Autodesk Fusion 360 part; units mm, degrees
sketch "rectangle" plane through (0, 0, 0) normal (0, 0, 1) x (1, 0, 0)
  line L0 (70, 35) -> (-70, 35)
  line L1 (-70, 35) -> (-70, -35)
  line L2 (-70, -35) -> (70, -35)
  line L3 (70, -35) -> (70, 35)
  line L4 (70, 35) -> (-70, -35) construction
  line L5 (-70, 35) -> (70, -35) construction
  dimension "d1" = 70
  dimension "d2" = 140
extrude "Extrude1" add sketch "rectangle" along normal blind 8
sketch "Sketch2" plane through (0, 0, 0) normal (0, 0, -1) x (1, 0, 0)
  line L0 (70, -35) -> (70, 35)
  line L1 (70, 35) -> (-70, 35)
  line L2 (-70, 35) -> (-70, -35)
  line L3 (-70, -35) -> (70, -35)
  line L4 (10, -45) -> (-10, -45)
  line L5 (-10, -45) -> (-10, 45)
  line L6 (-10, 45) -> (10, 45)
  line L7 (10, 45) -> (10, -45)
  line L8 (-6, 39) -> (-6, 21.0153)
  arc A0 (-6, 21.0153) -> (6, 21.0153) centre (0, 21.0153) ccw
  line L9 (6, 21.0153) -> (6, 39)
  arc A1 (6, 39) -> (-6, 39) centre (0, 39) ccw
  line L10 (0, 45) -> (0, 15.0153) construction
  dimension "d5" = 90
  dimension "d8" = 12
extrude "Extrude2" add sketch "Sketch2" along normal blind 8 contours L3 L4 L5 L7 | L1 L3 L5 L7 L8 A0 L9 | L1 L6 L7 L9 A1 | L1 L8 A0 L9 | L1 L8 L9 A1 | L1 L5 L6 L8 A1
sketch "Sketch3" plane through (0, 0, -8) normal (0, 0, -1) x (1, 0, 0)
  line L0 (10, 45) -> (-10, 45)
  line L1 (-10, 45) -> (-10, -45)
  line L2 (-10, -45) -> (10, -45)
  line L3 (10, -45) -> (10, 45)
  line L4 (10, -30) -> (10, 30)
  arc A0 (10, 30) -> (-10, 30) centre (0, 30) ccw
  line L5 (-10, 30) -> (-10, -30)
  arc A1 (-10, -30) -> (10, -30) centre (0, -30) ccw
  line L6 (0, -30) -> (0, 30) construction
extrude "Extrude3" add sketch "Sketch3" along normal blind 8 contours L1 L3 L4 A0 L5 A1
sketch "Sketch4" plane through (0, 0, -8) normal (0, 0, -1) x (1, 0, 0)
  arc A0 (-10, -30) -> (10, -30) centre (0, -30) ccw
  line L0 (-10, -45) -> (10, -45)
hole "Hole1" at (0, -30, -16) direction (0, 0, 1) diameter 10 depth 20 tip angle 118
hole "Hole2" at (0, 30, -16) direction (0, 0, 1) diameter 10 depth 20 tip angle 118
hole "Hole3" at (0, 0, -16) direction (0, 0, 1) diameter 10 depth 20 tip angle 118
fillet "Fillet1" radius 2 3 edges at (-10, -37.5, -8) (-10, -45, -4) (0, -45, -8)
fillet "Fillet2" radius 2 3 edges at (10, -45, -3) (10, -44.4142, -7.4142) (10, -36.5, -8)
fillet "Fillet3" radius 2 2 edges at (-10, 37.5, -8) (-10, 45, -4)
fillet "Fillet4" radius 2 2 edges at (10, 37.5, -8) (10, 45, -4)
Read the model definition and answer for the solid it produces. Units are mm, in the model's axes. A direction names the side the tool comes from. Round coordinates to 2 decimals unless told otherwise and drop trailing zeros. Write each loop counter-clockwise with the first axis right and the second up, starting at its lowest first coordinate (ties: lowest second). Pieces come first, ordered by that corner, then holes. Notation, with made-up numbers: (-39.75, 26) -> (-31.75, 26) arc R25 cw to (-31.75, 61) -> close; hole circle Ø10 at (23.25, 16). An arc over 180 degrees is marked (long way). Answer in a Markdown table with one row per item. Add a question column.
1) Find section A-A, the plane z = -11.5. Determine the outline of the cut face in (x, y), and give its area (3 significant figures).
2) Determine the mould class of faces 4 (the face through (-70, 0, 4)), 5 (the face through (0.04, -30.87, 6.48)), 6 (the face through (-7, -1, -16)) for opening direction X: pulls with the +X half, pulls with the -X half, needs draft (parallel to the pull), parting line crosses it, or undercut.
3) Given P1, Ø18, axis at x = -41, y = -16, coming from the -Z side; P2, Ø6.5, axis at x = 20, z = 2.5, coming from the -Y side; P3, Ø2.5, axis at x = 3.5, y = 40.5, coming from the -Z side; P4, Ø5, axis at y = -27, z = -7, coming from the -X side, each flat-ended and moving along its own axis, determine where each tip first touches the part or whether it passes through.
4) Find section B-B, the plane y = 21. Determine the outline of the cut face in (x, z).
5) Which of the six approach directions +Z, -Z, +X, -X, +Y, -Y give full straight-line access (tool end or side, diameter ignored) to faces 1 (the face through (0, -40, 0)), 2 (the face through (0, 40, 0)), 3 (the face through (0, -40, -12))?
6) Consider line 1 (Y direction, x = 0, z = -11.25); line 2 (Y direction, x = 0, z = -3); line 3 (X direction, y = -30, z = -8). Determine where each line is inside the solid, lowest interval first.
7) Find section D-D, the plane z = 2. Determine the outline of the cut face in (x, y), and give its area (3 significant figures).
8) Find section C-C, the plane x = 45.5. Determine the outline of the cut face in (y, z), and give its area (3 significant figures).
Findings below:
| question | item | result |
|---|---|---|
| 1 | outline | (-10, -30) arc R10 ccw to (10, -30) -> (10, 30) arc R10 ccw to (-10, 30) -> close; hole circle Ø10 at (0, -30); hole circle Ø10 at (0, 0); hole circle Ø10 at (0, 30) |
| 1 | area | 1,280 mm² |
| 2 | face 4 | pulls with the -X half |
| 2 | face 5 | undercut |
| 2 | face 6 | needs draft |
| 3 | P1 | z = 0 |
| 3 | P2 | y = -35 |
| 3 | P3 | z = -16 |
| 3 | P4 | x = -10 |
| 4 | outline | (-70, 0) -> (-10, 0) -> (-10, -16) -> (10, -16) -> (10, 0) -> (70, 0) -> (70, 8) -> (-70, 8) -> close |
| 5 | face 1 | +Z, +X, -X, -Y |
| 5 | face 2 | +Z, +X, -X, +Y |
| 5 | face 3 | -Z, -Y |
| 6 | line 1 | -40 to -35, -25 to -5, 5 to 25, 35 to 40 |
| 6 | line 2 | -45 to -35, -25 to -5, 5 to 25, 35 to 45 |
| 6 | line 3 | -10 to -5, 5 to 10 |
| 7 | outline | (-70, -35) -> (70, -35) -> (70, 35) -> (-70, 35) -> close; hole circle Ø10 at (0, -30); hole circle Ø10 at (0, 0); hole circle Ø10 at (0, 30) |
| 7 | area | 9,560 mm² |
| 8 | outline | (-35, 0) -> (35, 0) -> (35, 8) -> (-35, 8) -> close |
| 8 | area | 560 mm² |
